```python
from build123d import *

# Parameters (mm, degrees)
SKETCH1_R           = 2.5
BOSS_EXTRUDE3_DEPTH = 8


with BuildPart() as part:
    # Sketch1 → Boss-Extrude3 (new body)
    # profile 1 of 3: a face of its own
    with BuildSketch(Plane.XY):
        with BuildLine():
            ThreePointArc((30, 25), (33.535533906, 23.535533906), (35, 20))
            Line((35, 20), (35, -25))
            Line((35, -25), (-35, -25))
            Line((-35, -25), (-35, 20))
            ThreePointArc((-35, 20), (-33.535533906, 23.535533906), (-30, 25))
            Line((-30, 25), (30, 25))
        make_face()
        with Locations((14.25, 0)):
            Circle(SKETCH1_R, mode=Mode.SUBTRACT)
    # profile 2 of 3: a face of its own
    with BuildSketch(Plane.XY):
        with BuildLine():
            Line((-35, -10), (-35, 10))
            Line((-35, 10), (-55.909806165, 7.44461233))
            ThreePointArc((-55.909806165, 7.44461233), (-50.028760026, 5.615761134), (-47.5, 0))
            ThreePointArc((-47.5, 0), (-50.028760026, -5.615761134), (-55.909806165, -7.44461233))
            Line((-55.909806165, -7.44461233), (-35, -10))
        make_face()
    # profile 3 of 3: a face of its own
    with BuildSketch(Plane.XY):
        with BuildLine():
            ThreePointArc((-47.5, 0), (-50.028760026, 5.615761134), (-55.909806165, 7.44461233))
            ThreePointArc((-55.909806165, 7.44461233), (-62.5, 0), (-55.909806165, -7.44461233))
            ThreePointArc((-55.909806165, -7.44461233), (-50.028760026, -5.615761134), (-47.5, 0))
        make_face()
        with Locations((-52.5, 0)):
            Circle(SKETCH1_R, mode=Mode.SUBTRACT)
    extrude(amount=BOSS_EXTRUDE3_DEPTH)


solid = part.part
```
Source: CAD feature listing. Evaluate the final solid. Frame: model axes, mm. A direction names the side the tool comes from. Round coordinates to 2 decimals unless told otherwise and drop trailing zeros. Order: outer loops, then holes, each group sorted by start corner. A loop starts at its lowest first (then second) coordinate and runs counter-clockwise, first axis right, second up. Notation, with made-up numbers: (7, 57.25) -> (46, 57.25) arc R8 ccw to (46, 64.25) -> close; hole circle Ø8 at (-15.5, 71). An arc over 180 degrees is marked (long way). One line per item, written item: value. Start each with the question number.
Q1. Access query for faces 1 (the flat face through (-35, -18, 4)), 2 (the cylindrical face through (11.752, 0.11, 3.944)), 3 (the flat face through (-35, 15, 4)). Directions: +Z, -Z, +X, -X, +Y, -Y. A direction counts if a zero-diameter tool reaches every point of the face in a straight line with its end or side. Return the directions, or none.
Q2. Section query D-D (y = -17). Return the cut outline in (x, z).
Q3. Section query A-A (x = 14.25). Return the cut outline in (y, z).
Q4. Section query B-B (z = 2.75). Return the cut outline in (x, y), plus the area to 3 significant figures.
Q5. Section query C-C (y = 0). Return the cut outline in (x, z).
Q6. Pin query (flat end, axial travel): pin 1 (1 mm diameter, centred on y = -5.5, z = 2.5, fed in from -X); pin 2 (1 mm diameter, centred on y = 7, z = 7, fed in from -X); pin 3 (4.5 mm diameter, centred on x = -52.5, y = 0, fed in from -Z); pin 4 (1.5 mm diameter, centred on x = 1, y = -3, fed in from -Z). Return the tip coordinate at first contact, or that it passes through.
Q7. Material intervals for probe 1 along Y at (x, z) = (14.25, 3.5); probe 2 along Y at (x, z) = (-56, 3.5); probe 3 along Y at (x, z) = (-52.5, 3), sorted ascending.
Q8. Draft query along X for faces 4 (the cylindrical face through (-50.19, -0.96, 3.94)), 5 (the cylindrical face through (-34, 23, 4)), 6 (the flat face through (0, -25, 4)). Return one class per face: pulls with the +X half, pulls with the -X half, needs draft (parallel to the pull), parting line crosses it, or undercut.
Findings below:
1. face 1: +Z, -Z, -X, -Y
1. face 2: +Z, -Z
1. face 3: +Z, -Z, -X, +Y
2. outline: (-35, 0) -> (35, 0) -> (35, 8) -> (-35, 8) -> close
3. outline: (-25, 0) -> (-2.5, 0) -> (-2.5, 8) -> (-25, 8) -> close; (2.5, 0) -> (25, 0) -> (25, 8) -> (2.5, 8) -> close
4. outline: (-55.91, -7.44) -> (-35, -10) -> (-35, -25) -> (35, -25) -> (35, 20) arc R5 ccw to (30, 25) -> (-30, 25) arc R5 ccw to (-35, 20) -> (-35, 10) -> (-55.91, 7.44) arc R7.5 ccw to start; hole circle Ø5 at (-52.5, 0); hole circle Ø5 at (14.25, 0)
4. area: 3,890 mm²
5. outline: (-62.5, 0) -> (-55, 0) -> (-55, 8) -> (-62.5, 8) -> close; (-50, 0) -> (11.75, 0) -> (11.75, 8) -> (-50, 8) -> close; (16.75, 0) -> (35, 0) -> (35, 8) -> (16.75, 8) -> close
6. pin 1: x = -60.59
6. pin 2: x = -58.74
6. pin 3: through
6. pin 4: z = 0
7. probe 1: -25 to -2.5, 2.5 to 25
7. probe 2: -7.43 to 7.43
7. probe 3: -7.86 to -2.5, 2.5 to 7.86
8. face 4: undercut
8. face 5: pulls with the -X half
8. face 6: needs draft
